```python
from build123d import *

# Parameters (mm, degrees)
BOSS_EXTRUDE1_DEPTH     = 5
SKETCH2_W               = 10
SKETCH2_H               = 5
BOSS_EXTRUDE2_DEPTH     = 15.5
BOSS_EXTRUDE3_DEPTH     = 6.5
CHAMFER1_SIZE           = 10
CHAMFER2_SIZE           = 5
CUT_EXTRUDE1_DEPTH      = 5
CUT_EXTRUDE1_DEPTH_BACK = 2
SKETCH4_R               = 3.75
SKETCH5_W               = 13.5
SKETCH5_H               = 30
CUT_EXTRUDE2_DEPTH      = 2
CHAMFER3_SIZE           = 1.5
SKETCH6_R               = 2
CUT_EXTRUDE4_DEPTH      = 44.794976881
FILLET1_R               = 3


with BuildPart() as part:
    # Sketch1 → Boss-Extrude1 (new body)
    with BuildSketch(Plane.XY):
        with BuildLine():
            Line((0, 24.45), (0, 30))
            Line((0, 30), (17, 30))
            Line((17, 30), (17, 25))
            Line((17, 25), (7, 25))
            Line((7, 25), (7, 0))
            Line((7, 0), (0, 0))
            Line((0, 0), (0, 5.95))
            ThreePointArc((0, 5.95), (1.75, 7.7), (0, 9.45))
            Line((0, 9.45), (0, 20.95))
            ThreePointArc((0, 20.95), (1.75, 22.7), (0, 24.45))
        make_face()
    extrude(amount=BOSS_EXTRUDE1_DEPTH)

    # Sketch2 → Boss-Extrude2 (add)
    with BuildSketch(Plane.XY.offset(5)):
        with Locations((12, 27.5)):
            Rectangle(SKETCH2_W, SKETCH2_H)
    extrude(amount=BOSS_EXTRUDE2_DEPTH)

    # Sketch3 → Boss-Extrude3 (add)
    with BuildSketch(Plane.XY.offset(20.5)):
        Polygon((7, 0), (7, 25), (17, 25), (17, 30), (0, 30), (0, 0), align=None)
    extrude(amount=BOSS_EXTRUDE3_DEPTH)

    # Chamfer1
    chamfer1_edges = [part.edges().sort_by_distance(p)[0] for p in [
        (7, 25, 2.5),
        (7, 25, 23.75),
    ]]
    chamfer(chamfer1_edges, length=CHAMFER1_SIZE - 0.0001)  # a hair under: the kernel refuses the full size

    # Chamfer2
    chamfer2_edges = [part.edges().sort_by_distance(p)[0] for p in [
        (11.99995, 25, 5),
        (11.99995, 25, 20.5),
    ]]
    chamfer(chamfer2_edges, length=CHAMFER2_SIZE)

    # Sketch4 → Cut-Extrude1 (cut, two sides: drawn at the far end of the back side and taken through both)
    with BuildSketch(Plane.XZ.offset(-25).offset(-CUT_EXTRUDE1_DEPTH_BACK)):
        with Locations(Location((12, 12.75, 0), (0, 0, 132.833428066))):
            Circle(SKETCH4_R)
    extrude(amount=CUT_EXTRUDE1_DEPTH + CUT_EXTRUDE1_DEPTH_BACK, mode=Mode.SUBTRACT)

    # Mirror1: part across plane


with BuildPart() as part_1:
    add(part.part)
    add(part.part.mirror(Plane(origin=(0, 30, 27), x_dir=(0, 0, 1), z_dir=(1, 0, 0))))

    # Sketch5 → Cut-Extrude2 (cut)
    with BuildSketch(Plane.XY.offset(27)):
        with Locations((-10.25, 15)):
            Rectangle(SKETCH5_W, SKETCH5_H)
        with Locations((10.25, 15)):
            Rectangle(SKETCH5_W, SKETCH5_H)
    extrude(amount=-CUT_EXTRUDE2_DEPTH, mode=Mode.SUBTRACT)

    # Chamfer3
    chamfer3_edges = [part_1.edges().sort_by_distance(p)[0] for p in [
        (0, 9.45, 0),
        (0, 24.45, 0),
    ]]
    chamfer(chamfer3_edges, length=CHAMFER3_SIZE)

    # Sketch6 → Cut-Extrude4 (cut, through all)
    with BuildSketch(Plane(origin=(0, 30, 0), x_dir=(1, 0, 0), z_dir=(0, 1, 0))):
        with Locations((-7, -12.75)):
            Circle(SKETCH6_R)
    extrude(amount=-CUT_EXTRUDE4_DEPTH, mode=Mode.SUBTRACT)

    # Fillet1
    fillet1_edges = [part_1.edges().sort_by_distance(p)[0] for p in [
        (-7, 27.5, 14.75),
        (-7, 27.5, 10.75),
    ]]
    fillet(fillet1_edges, radius=FILLET1_R)


solid = part_1.part
```
Here's how the part is built. I have some questions about the finished solid (model axes, mm). A direction names the side the tool comes from. Round coordinates to 2 decimals unless told otherwise and drop trailing zeros. Write each loop counter-clockwise with the first axis right and the second up, starting at its lowest first coordinate (ties: lowest second). Pieces come first, ordered by that corner, then holes.
Q1. If we section it at D-D on y = 3: Write out the boundary of the cut face in (x, z).
Q2. If we section it at C-C on y = 28.25: Write out the boundary of the cut face in (x, z).
Q3. If we section it at A-A on x = 4: Write out the boundary of the cut face in (y, z), plus the area to 3 significant figures.
Q4. If we mould it in two halves opening along X, with no side actions, what happens to faces 6 (the flat face through (0, 0, 23)), 7 (the flat face through (-7, 26, 7)), 8 (the flat face through (13, 21, 4))? For each: +X half, -X half, draft (parallel to the pull), parting line (faces both ways), or undercut.
Q5. Please list where these lines run through material, in increasing order: probe 1 along X at (y, z) = (25.8, 12.75); probe 2 along Z at (x, y) = (-12, 25.4); probe 3 along Z at (x, y) = (-6.5, 10.25).
Q6. If we section it at B-B on z = 2: Give the number of separate pieces and of enclosed holes in the cut face, plus the area to 3 significant figures.
Q7. Which directions (+Z, -Z, +X, -X, +Y, -Y) give clear straight access to the entire face, cutting with the end or side of a thin tool? Please do faces 1 (the flat face through (7, 8, 2)), 2 (the flat face through (-7, 8, 2)), 3 (the cylindrical face through (-7.308, 27.613, 10.074)), 4 (the flat face through (10.8, 22.5, 18)), 5 (the flat face through (-9, 22, 25)).
Q8. Will these pins go through, and if not, where does the flat tip stop? P1, Ø15, axis at x = 12, y = 9, coming from the +Z side; P2, Ø3.5, axis at y = 5.5, z = 22.5, coming from the +X side; P3, Ø1.1, axis at x = -9, z = 10.5, coming from the -Y side.
Answer below:
1. outline: (-7, 0) - (7, 0) - (7, 5) - (-7, 5) - close; (-7, 20.5) - (7, 20.5) - (7, 25) - (3.5, 25) - (3.5, 27) - (-3.5, 27) - (-3.5, 25) - (-7, 25) - close
2. outline: (-17, 0) - (17, 0) - (17, 25) - (3.5, 25) - (3.5, 27) - (-3.5, 27) - (-3.5, 25) - (-17, 25) - close; hole (-8.2, 11.15) arc R3 cw to (-7, 8.75) - (-7, 5) - (7, 5) - (7, 20.5) - (-7, 20.5) - (-7, 16.75) arc R3 cw to (-8.2, 14.35) arc R2 ccw to start
3. outline: (0, 0) - (30, 0) - (30, 5) - (0, 5) - close; (0, 20.5) - (30, 20.5) - (30, 25) - (0, 25) - close
3. area: 285 mm2
4. face 6: draft
4. face 7: undercut
4. face 8: +X half
5. probe 1: x = -17 to -15.75, 7 to 8.25, 15.75 to 17
5. probe 2: z = 0 to 9, 16.5 to 25
5. probe 3: z = 0 to 5, 20.5 to 25
6. separate pieces: 1
6. enclosed holes: 2
6. area: 601 mm2
7. face 1: +Z, -Z, +X, -Y
7. face 2: +Z, -Z, -X, -Y
7. face 3: +Y, -Y
7. face 4: +X, -X, -Y
7. face 5: +Z, -X, +Y, -Y
8. P1: stops at z = 25
8. P2: stops at x = 7
8. P3: stops at y = 24.95
